Part print with two shaded views. Sizes in mm from the minimum x, y, z corner. Coordinates: 2 decimals unless noted, no trailing zeros. Loops run counter-clockwise (first coordinate to the right, second up) from the corner with the lowest first, then second, coordinate; pieces in that order, holes last.
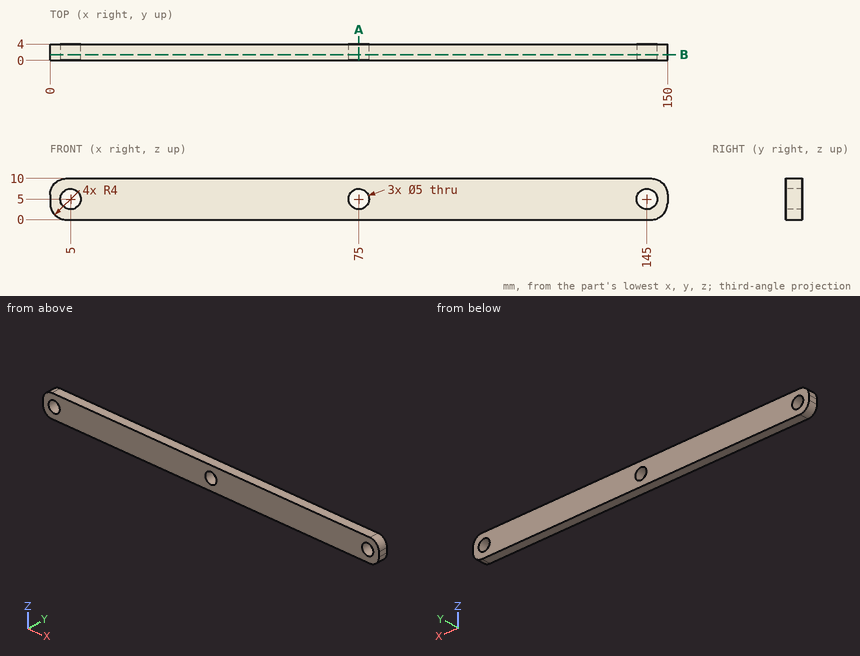
Q1. Slice it at A-A (x = 75). List the corners of the cut face in (y, z), and give its area (3 significant figures).
Answers:
outline: (0, 0) - (4, 0) - (4, 2.5) - (0, 2.5) - close; (0, 7.5) - (4, 7.5) - (4, 10) - (0, 10) - close
area: 20.0 mm2
Q2. Slice it at B-B (y = 1.4). List the corners of the cut face in (x, z).
Answers:
outline: (0, 4) arc R4 ccw to (4, 0) - (146, 0) arc R4 ccw to (150, 4) - (150, 6) arc R4 ccw to (146, 10) - (4, 10) arc R4 ccw to (0, 6) - close; hole circle Ø5 at (5, 5); hole circle Ø5 at (75, 5); hole circle Ø5 at (145, 5)
Q3. Drill centre lines: line 1 (Z direction, x = 5, y = 1.65); line 2 (X direction, y = 3.5, z = 4.25); line 3 (X direction, y = 0.2, z = 3.5). Where is each one in solid material? Low to high.
Answers:
line 1: z = 0 to 2.5, 7.5 to 10
line 2: x = 0 to 2.62, 7.38 to 72.62, 77.38 to 142.62, 147.38 to 150
line 3: x = 0.03 to 3, 7 to 73, 77 to 143, 147 to 149.97
Q4. Flat gauge pin, fed straight in: P1, Ø1.5, axis at y = 1.5, z = 2, coming from the -X side. Where does the tip first touch, or does it go through?
Answers:
P1: stops at x = 0.2
